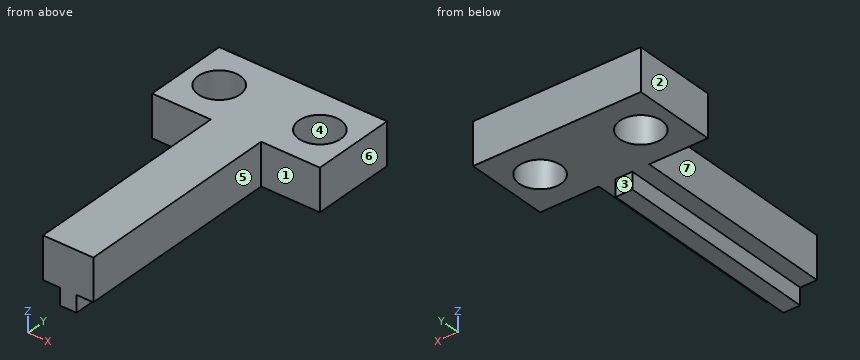
from build123d import *

# Parameters (mm, degrees)
SKETCH_W     = 20
SKETCH_H     = 10
SKETCH_R     = 2.5
PAD_DEPTH    = 5
SKETCH001_W  = 6
SKETCH001_H  = 5
PAD001_DEPTH = 25
SKETCH002_W  = 2
SKETCH002_H  = 25
PAD002_DEPTH = 2


with BuildPart() as part:
    # Sketch → Pad (new body)
    with BuildSketch(Plane.XY):
        Rectangle(SKETCH_W, SKETCH_H)
        with Locations((-6, 0)):
            Circle(SKETCH_R, mode=Mode.SUBTRACT)
        with Locations((6, 0)):
            Circle(SKETCH_R, mode=Mode.SUBTRACT)
    extrude(amount=PAD_DEPTH)

    # Sketch001 → Pad001 (new body)
    with BuildSketch(Plane.XZ.offset(5)):
        with Locations((0, 2.5)):
            Rectangle(SKETCH001_W, SKETCH001_H)
    extrude(amount=PAD001_DEPTH)

    # Sketch002 → Pad002 (new body)
    with BuildSketch(Plane(origin=(0, 0, 0), x_dir=(1, 0, 0), z_dir=(0, 0, -1))):
        with Locations((0, 17.5)):
            Rectangle(SKETCH002_W, SKETCH002_H)
    extrude(amount=PAD002_DEPTH)


solid = part.part
Geometry: final body of the model. Coordinates: model frame, mm. Face numbers are marked on the shaded views. A direction names the side the tool comes from. Round coordinates to 2 decimals unless told otherwise and drop trailing zeros. Loops run counter-clockwise (first coordinate to the right, second up) from the corner with the lowest first, then second, coordinate; pieces in that order, holes last. Notation, with made-up numbers: (-29, 0) - (26, 0) arc R16 cw to (26, 30) - close; hole circle Ø9 at (33, 27.25). An arc over 180 degrees is marked (long way). Write each question's results on one line, items separated by ' | '. Start each with the question number.
1) Cut plane B-B on x = -6. Return loops of the section in (y, z), then the cut area to 3 significant figures.
2) Line query: probe 1 along Y at (x, z) = (-6, 2.5); probe 2 along X at (y, z) = (1.5, 3.25); probe 3 along Z at (x, y) = (3, -3). Output: solid intervals per line, ascending. Write a range as [from, to].
3) Cut plane C-C on z = 4.25. Return loops of the section in (x, y).
4) Mould query, pull axis Y, two halves, no side actions, for the marked faces 1, 2, 3 and 4. Classes: released by +Y, released by -Y, zero draft, split by the parting line, or undercut.
5) Cut plane A-A on y = 0. Return loops of the section in (x, z).
6) Access query for the marked faces 5, 6 and 7. Directions: +Z, -Z, +X, -X, +Y, -Y. A direction counts if a zero-diameter tool reaches every point of the face in a straight line with its end or side. Return the directions, or none.
7) Cut plane D-D on y = -13. Return loops of the section in (x, z), then the cut area to 3 significant figures.
8) First-contact query: P1, Ø10, axis at x = -6, y = -9.5, coming from the +Z side; P2, Ø4, axis at x = 7.5, z = 1.5, coming from the -Y side; P3, Ø8, axis at x = 6, y = 0, coming from the -Z side; P4, Ø4, axis at y = -23.5, z = 1, coming from the +X side. Flat tips, straight axial feed; report the tip coordinate or a pass-through.
Verdict:
1) outline: (-5, 0) - (-2.5, 0) - (-2.5, 5) - (-5, 5) - close; (2.5, 0) - (5, 0) - (5, 5) - (2.5, 5) - close | area: 25.0 mm2
2) probe 1: y = [-5, -2.5], [2.5, 5] | probe 2: x = [-10, -8], [-4, 4], [8, 10] | probe 3: z = [0, 5]
3) outline: (-10, -5) - (-3, -5) - (-3, -30) - (3, -30) - (3, -5) - (10, -5) - (10, 5) - (-10, 5) - close; hole circle Ø5 at (-6, 0); hole circle Ø5 at (6, 0)
4) face 1: released by -Y | face 2: zero draft | face 3: released by +Y | face 4: undercut
5) outline: (-10, 0) - (-8.5, 0) - (-8.5, 5) - (-10, 5) - close; (-3.5, 0) - (3.5, 0) - (3.5, 5) - (-3.5, 5) - close; (8.5, 0) - (10, 0) - (10, 5) - (8.5, 5) - close
6) face 5: +Z, -Z, +X, -Y | face 6: +Z, -Z, +X, +Y, -Y | face 7: +Z, -Z, -X, -Y
7) outline: (-3, 0) - (-1, 0) - (-1, -2) - (1, -2) - (1, 0) - (3, 0) - (3, 5) - (-3, 5) - close | area: 34.0 mm2
8) P1: stops at z = 5 | P2: stops at y = -5 | P3: stops at z = 0 | P4: stops at x = 3
